The model under review builds one solid part; all positions refer to its coordinate system, in mm. Face numbers are marked on the shaded views. A direction names the side the tool comes from. Give positions to 0.01 mm unless a question says otherwise; leave off trailing zeros. Order: outer loops, then holes, each group sorted by start corner. A loop starts at its lowest first (then second) coordinate and runs counter-clockwise, first axis right, second up. Notation, with made-up numbers: M -22.5,73 L 3.5,73 A34 ccw 3.5,104 Z; hole C 67.25,83.25 d6. An arc over 180 degrees is marked long. One line per question, with ' | ' between items. Start each with the question number.
1. We need section B-B on z = 0. Write out the cut boundary in (x, y), then the cut area to 3 significant figures.
2. We need section A-A on y = 11. Write out the cut boundary in (x, z), then the cut area to 3 significant figures.
3. The part is to be moulded in two halves that separate along X. For the marked faces 1, 2 and 3, say which applies: +X half, -X half, draft (parallel to the pull), parting line (faces both ways), or undercut.
4. We need section C-C on y = 2.2. Write out the cut boundary in (x, z), then the cut area to 3 significant figures.
5. Insertion check: P1, Ø1.8, axis at y = 4, z = -1.5, coming from the -X side; P2, Ø6, axis at y = 10.5, z = 2.5, coming from the -X side; P3, Ø1.5, axis at x = 4.5, z = 4.5, coming from the +Y side. Each pin has a flat end and moves straight along its axis. Give the tip position at first contact, or say it passes through.
6. We need section D-D on x = 23.5. Write out the cut boundary in (y, z), then the cut area to 3 significant figures.
7. For the marked faces 4, 5 and 6, list the 3-axis set-ups (+Z, -Z, +X, -X, +Y, -Y) from which the entire face can be reached by the end or side of a thin tool; tool diameter is ignored.
8. Wall thickness on L1, parallel to Y at x = 2.5, z = -0.75; L2, parallel to Y at x = 15.5, z = -5.5; L3, parallel to X at y = 12.25, z = -4.75: over which ranges is each line inside the solid? List them lowest first.
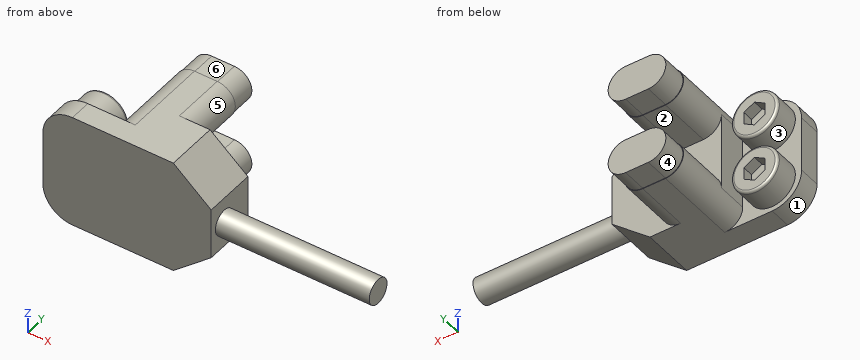
Autodesk Inventor part; units mm, degrees
ref_plane "gth4_sensor_XY" through (0, 0, 0) normal (1, 0, 0) x (0, 0, -1)
ref_plane "gth4_sensor_YZ" through (0, 0, 0) normal (0, 0, -1) x (0, 1, 0)
ref_plane "gth4_sensor_ZX" through (0, 0, 0) normal (0, 1, 0) x (1, 0, 0)
sketch "Sketch_1" plane through (0, 0, 0) normal (0, 0, 1) x (1, 0, 0)
  line L0 (0, 2.6) -> (0, 0)
  line L1 (0, 0) -> (20, 0)
  line L2 (20, 0) -> (20, 6.2)
  line L3 (20, 6.2) -> (7, 6.2)
  line L4 (7, 6.2) -> (7, 2.6)
  line L5 (7, 2.6) -> (0, 2.6)
extrude "Extrusion1" add sketch "Sketch_1" along normal mid plane 13.6
fillet "Fillet1" radius 3.5 2 edges at (0, 1.3, 6.8) (0, 1.3, -6.8)
fillet "Fillet2" radius 2.15 2 edges at (7, 4.4, 6.8) (7, 4.4, -6.8)
sketch "Sketch_4" plane through (20, 0, 0) normal (1, 0, 0) x (0, 0, -1)
  circle A0 centre (0, 2.2) radius 1.5
extrude "Extrusion2" add sketch "Sketch_4" along normal blind 18.3
sketch "Sketch_7" plane through (0, 0, 3.5) normal (0, 0, 1) x (1, 0, 0)
  line L0 (3.5, 2.6) -> (3.5, 5.6)
  line L1 (3.5, 5.6) -> (5.95, 5.6)
  arc A0 (6.25, 5.3) -> (5.95, 5.6) centre (5.95, 5.3) ccw
  line L2 (6.25, 5.3) -> (6.25, 2.6)
  line L3 (6.25, 2.6) -> (3.5, 2.6)
  line L4 (3.5, 2.6) -> (3.5, 5.6)
revolve "Revolution1" add sketch "Sketch_7" angle 360 about axis through (3.5, 2.6, 3.5) along (0, -1, 0)
pattern_linear "Rectangular Pattern1" count 2 spacing 7 along (0, 0, -1) of "Revolution1"
sketch "Sketch_9" plane through (0, 5.6, 0) normal (0, 1, 0) x (1, 0, 0)
  line L0 (2.25, -4.2217) -> (3.5, -4.9434)
  line L1 (3.5, -4.9434) -> (4.75, -4.2217)
  line L2 (4.75, -4.2217) -> (4.75, -2.7783)
  line L3 (4.75, -2.7783) -> (3.5, -2.0566)
  line L4 (3.5, -2.0566) -> (2.25, -2.7783)
  line L5 (2.25, -2.7783) -> (2.25, -4.2217)
extrude "Extrusion3" cut sketch "Sketch_9" against normal blind 1.3
pattern_linear "Rectangular Pattern2" count 2 spacing 7 along (0, 0, -1) of "Extrusion3"
sketch "__1" plane through (0, 6.2, 0) normal (0, 1, 0) x (1, 0, 0)
  arc A0 (9.15, -2.5) -> (9.15, -6.8) centre (9.15, -4.65) ccw
  line L0 (9.15, -6.8) -> (11.85, -6.8)
  arc A1 (11.85, -6.8) -> (11.85, -2.5) centre (11.85, -4.65) ccw
  line L1 (11.85, -2.5) -> (9.15, -2.5)
extrude "Extrusion4" add sketch "__1" along normal blind 6.4
sketch "__2" plane through (0, 6.2, 0) normal (0, 1, 0) x (1, 0, 0)
  arc A0 (9.15, 6.8) -> (9.15, 2.5) centre (9.15, 4.65) ccw
  line L0 (9.15, 2.5) -> (11.85, 2.5)
  arc A1 (11.85, 2.5) -> (11.85, 6.8) centre (11.85, 4.65) ccw
  line L1 (11.85, 6.8) -> (9.15, 6.8)
extrude "Extrusion5" add sketch "__2" along normal blind 6.4
sketch "__3" plane through (0, 12.6, 0) normal (0, 1, 0) x (1, 0, 0)
  arc A0 (9.15, -2.57) -> (9.15, -6.73) centre (9.15, -4.65) ccw
  line L0 (9.15, -6.73) -> (11.85, -6.73)
  arc A1 (11.85, -6.73) -> (11.85, -2.57) centre (11.85, -4.65) ccw
  line L1 (11.85, -2.57) -> (9.15, -2.57)
extrude "Extrusion6" add sketch "__3" along normal blind 2.9
sketch "__4" plane through (0, 12.6, 0) normal (0, 1, 0) x (1, 0, 0)
  arc A0 (9.15, 6.73) -> (9.15, 2.57) centre (9.15, 4.65) ccw
  line L0 (9.15, 2.57) -> (11.85, 2.57)
  arc A1 (11.85, 2.57) -> (11.85, 6.73) centre (11.85, 4.65) ccw
  line L1 (11.85, 6.73) -> (9.15, 6.73)
extrude "Extrusion7" add sketch "__4" along normal blind 2.9
sketch "__5" plane through (0, 0, 0) normal (0, 1, 0) x (-1, 0, 0)
  line L0 (-15.5, 6.8) -> (-20, 6.8)
  line L1 (-20, 6.8) -> (-20, 3.0241)
  line L2 (-20, 3.0241) -> (-15.5, 6.8)
extrude "Extrusion8" cut sketch "__5" along normal blind 10
sketch "__6" plane through (0, 0, 0) normal (0, 1, 0) x (-1, 0, 0)
  line L0 (-15.5, -6.8) -> (-20, -3.0241)
  line L1 (-20, -3.0241) -> (-20, -6.8)
  line L2 (-20, -6.8) -> (-15.5, -6.8)
extrude "Extrusion9" cut sketch "__6" along normal blind 10
ref_plane "gth4_sensor_XY" through (0, 0, 0) normal (1, 0, 0) x (0, 0, -1)
ref_plane "gth4_sensor_YZ" through (0, 0, 0) normal (0, 0, -1) x (0, 1, 0)
ref_plane "gth4_sensor_ZX" through (0, 0, 0) normal (0, 1, 0) x (1, 0, 0)
properties part number "ETH2-14-sensor"
Entries:
1) outline: M 0,0 L 20,0 L 20,0.7 L 38.3,0.7 L 38.3,3.7 L 20,3.7 L 20,6.2 L 7,6.2 L 7,2.6 L 0,2.6 Z | area: 154 mm^2
2) outline: M 9.15,-6.8 L 11.85,-6.8 A2.15 ccw 11.85,-2.5 L 9.15,-2.5 A2.15 ccw Z; M 9.15,2.5 L 11.85,2.5 A2.15 ccw 11.85,6.8 L 9.15,6.8 A2.15 ccw Z | area: 52.3 mm^2
3) face 1: -X half | face 2: draft | face 3: undercut
4) outline: M 0,-3.3 A3.5 ccw 3.5,-6.8 L 15.5,-6.8 L 20,-3.02 L 20,-1.5 L 38.3,-1.5 L 38.3,1.5 L 20,1.5 L 20,3.02 L 15.5,6.8 L 3.5,6.8 A3.5 ccw 0,3.3 Z | area: 305 mm^2
5) P1: stops at x = 0.98 | P2: stops at x = 7 | P3: stops at y = 5.6
6) outline: C 2.2,0 d3 | area: 7.07 mm^2
7) face 4: -X, +Y | face 5: +X, +Y | face 6: +Z, +X, -X, +Y
8) L1: y = 0 to 2.6 | L2: y = 0 to 6.2 | L3: x = 7 to 14
